Autodesk Fusion 360 part; units mm, degrees
sketch "Sketch1" plane through (0, 0, 0) normal (0, 1, 0) x (1, 0, 0)
  line L0 (0, 0) -> (0, -408.4277) construction
  line L1 (0, -660.4) -> (0, -355.6)
  line L2 (0, -355.6) -> (254, -355.6)
  line L3 (254, -355.6) -> (254, 0)
  line L4 (254, 0) -> (317.5, 0)
  line L5 (317.5, 0) -> (317.5, -406.4)
  line L6 (317.5, -406.4) -> (292.1, -406.4)
  line L7 (292.1, -406.4) -> (292.1, -431.8)
  line L8 (292.1, -431.8) -> (317.5, -431.8)
  line L9 (317.5, -431.8) -> (317.5, -469.9)
  line L10 (317.5, -469.9) -> (292.1, -469.9)
  line L11 (292.1, -469.9) -> (292.1, -495.3)
  line L12 (292.1, -495.3) -> (317.5, -495.3)
  line L13 (317.5, -495.3) -> (317.5, -533.4)
  line L14 (317.5, -533.4) -> (292.1, -533.4)
  line L15 (292.1, -533.4) -> (292.1, -558.8)
  line L16 (292.1, -558.8) -> (317.5, -558.8)
  line L17 (317.5, -558.8) -> (317.5, -609.6)
  arc A0 (0, -660.4) -> (317.5, -609.6) centre (0, 357.1875) ccw
  line L18 (0, -660.4) -> (-298.2009, -660.4) construction
  dimension "d1" = 508
  dimension "d2" = 635
  dimension "d3" = 355.6
  dimension "d4" = 406.4
  dimension "d5" = 25.4
  dimension "d6" = 25.4
  dimension "d7" = 38.1
  dimension "d8" = 50.8
  dimension "d9" = 660.4
revolve "Revolve1" add sketch "Sketch1" angle 360 about axis through (0, 0, 0) along (0, 0, 1)
ref_plane "WorkPlane1" through (317.5, 0, 0) normal (1, 0, 0) x (0, 1, 0)
sketch "Sketch2" plane through (317.5, 0, 0) normal (1, 0, 0) x (0, 1, 0)
  circle A0 centre (0, 228.6) radius 120.65
  dimension "d12" = 241.3
  dimension "d13" = 228.6
extrude "Extrude1" cut sketch "Sketch2" against normal blind 38.1
sketch "Sketch3" plane through (279.4, 0, 0) normal (1, 0, 0) x (0, 1, 0)
  circle A0 centre (0, 228.6) radius 120.65
  circle A1 centre (0, 228.6) radius 88.9
  dimension "d16" = 177.8
extrude "Extrude2" cut sketch "Sketch3" against normal blind 127 contours A1
mirror "Mirror1" about plane through (0, 0, 0) normal (1, 0, 0) of "Extrude1", "Extrude2"
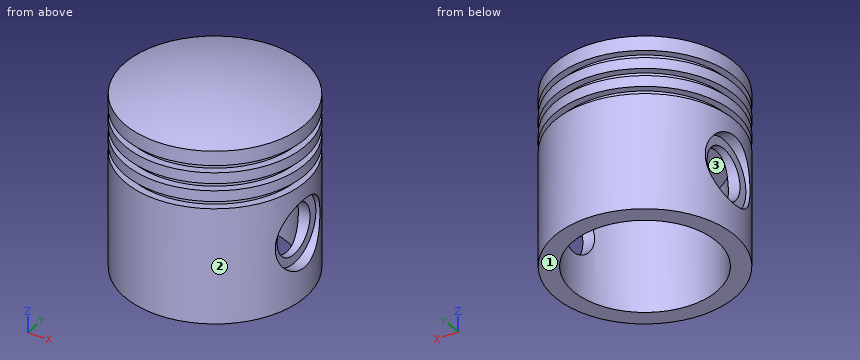
Build history of the part. All positions in model axes, mm. Face numbers are marked on the shaded views. Round coordinates to 2 decimals unless told otherwise and drop trailing zeros. Order: outer loops, then holes, each group sorted by start corner. A loop starts at its lowest first (then second) coordinate and runs counter-clockwise, first axis right, second up. Notation, with made-up numbers: (3.25, 71.25) - (48.25, 71.25) arc R20 cw to (48.25, 109.25) - close; hole circle Ø7 at (-21, -31.5). An arc over 180 degrees is marked (long way). Use a Markdown table: item, result.
1) Saw through at B-B on z = 274. Write the cut outline in (x, y), and give its area (3 significant figures).
Recorded:
| item | result |
|---|---|
| outline | (-297.17, -111.78) arc R317.5 ccw to (297.17, -111.78) - (279.4, -111.78) - (279.4, -76.43) - (242.23, -76.43) arc R254 cw to (-242.23, -76.43) - (-279.4, -76.43) - (-279.4, -111.78) - close; (-297.17, 111.78) - (-279.4, 111.78) - (-279.4, 76.43) - (-242.23, 76.43) arc R254 cw to (242.23, 76.43) - (279.4, 76.43) - (279.4, 111.78) - (297.17, 111.78) arc R317.5 ccw to start |
| area | 91,000 mm² |
2) Saw through at C-C on y = 0. Give the number of separate pieces and of enclosed holes in the cut face, and give its area (3 significant figures).
Recorded:
| item | result |
|---|---|
| separate pieces | 3 |
| enclosed holes | 0 |
| area | 197,000 mm² |
3) Flat gauge pins, fed straight in: pin 1 Ø4 at (x, y) = (-240, -167.5) entering from -Z; pin 2 Ø10 at (x, z) = (-135.5, 459) entering from -Y; pin 3 Ø8 at (x, z) = (189.5, 442) entering from +Y; pin 4 Ø1.5 at (x, z) = (-252.5, 157.5) entering from +Y. Where does each tip first touch, or does it go through?
Recorded:
| item | result |
|---|---|
| pin 1 | stops at z = 0 |
| pin 2 | stops at y = -289.44 |
| pin 3 | stops at y = 257.67 |
| pin 4 | stops at y = 193.46 |
4) Wall check: L1, parallel to Y at x = 0, z = 205; L2, parallel to X at y = -209, z = 164; L3, parallel to X at y = 208, z = 42.5. Give the ranges that are in metal, low to high.
Recorded:
| item | result |
|---|---|
| L1 | y = -317.5 to -254, 254 to 317.5 |
| L2 | x = -239.01 to -144.34, 144.34 to 239.01 |
| L3 | x = -239.88 to -145.78, 145.78 to 239.88 |
5) Pull direction X, two halves, no side cores. Call the marked faces 1, 2 and 3: pulls with the +X half, pulls with the -X half, needs draft (parallel to the pull), parting line crosses it, or undercut.
Recorded:
| item | result |
|---|---|
| face 1 | needs draft |
| face 2 | parting line crosses it |
| face 3 | undercut |
